```python
from build123d import *

# Parameters (mm, degrees)
F1_DEPTH    = 9.525
F3_DEPTH    = 33.02
F4_T1_DEPTH = 49.53
F6_DEPTH    = 10.16
F7_R        = 3.175
F8_DEPTH    = 25.4
F10_DEPTH   = 25.4


# Not quite as in the source:
# - a fillet or chamfer that OpenCascade refuses, or shapes differently, is made with other operations: its cross-section is extruded or revolved along the edge and cut away or added


with BuildPart() as f1:
    # F0 (on Front) → F1 (new body, symmetric)
    with BuildSketch(Plane.XZ):
        Polygon((-5.715, 0), (0, 0), (0, 1.778), (21.59, 1.778), (21.59, 0), (27.305, 0), (27.305, 4.572), (-5.715, 4.572), align=None)
    extrude(amount=F1_DEPTH, both=True)

    # F2 (on face) → F3 (cut)
    with BuildSketch(Plane.YZ.offset(27.305)):
        Polygon((-2.286, 0), (0, 0), (2.286, 0), (2.286, 1.778), (0, 1.778), (-2.286, 1.778), align=None)
    extrude(amount=-F3_DEPTH, mode=Mode.SUBTRACT)

    # F4: fillet of radius 3.302 on 2 edges, made by hand

    # F4_s2 → F4_t1 (cut)
    with BuildSketch(Plane.YZ.offset(-13.97)):
        with BuildLine():
            ThreePointArc((-6.223, 4.572), (-8.5578665915, 3.6048665915), (-9.525, 1.27))
            Line((-9.525, 1.27), (-9.525, 4.572))
            Line((-9.525, 4.572), (-6.223, 4.572))
        make_face()
        with BuildLine():
            ThreePointArc((9.525, 1.27), (8.5578665915, 3.6048665915), (6.223, 4.572))
            Line((6.223, 4.572), (9.525, 4.572))
            Line((9.525, 4.572), (9.525, 1.27))
        make_face()
    extrude(amount=F4_T1_DEPTH, mode=Mode.SUBTRACT)

    # F5 (on face) → F6 (join)
    with BuildSketch(Plane.XY.offset(4.572)):
        Polygon((-5.715, 3.429), (-5.715, 0), (-5.715, -3.429), (5.969, -3.429), (5.969, 3.429), align=None)
        Polygon((27.305, 0), (27.305, 3.429), (15.621, 3.429), (15.621, -3.429), (27.305, -3.429), align=None)
    extrude(amount=F6_DEPTH)

    # F7 (on face) → F8 (cut)
    with BuildSketch(Plane.XZ.offset(3.429)):
        Polygon((-5.715, 14.732), (-5.715, 8.382), (0.127, 14.732), align=None)
        with Locations((0, 8.382)):
            Circle(F7_R)
    extrude(amount=-F8_DEPTH, mode=Mode.SUBTRACT)

    # F9 (on face) → F10 (cut)
    with BuildSketch(Plane.XZ.offset(3.429)):
        Polygon((27.305, 14.732), (20.955, 14.732), (27.305, 8.382), align=None)
    extrude(amount=-F10_DEPTH, mode=Mode.SUBTRACT)


solid = f1.part
```
Build history of the part. All positions in model axes, mm. A direction names the side the tool comes from. Give positions to 0.01 mm unless a question says otherwise; leave off trailing zeros. Order: outer loops, then holes, each group sorted by start corner. A loop starts at its lowest first (then second) coordinate and runs counter-clockwise, first axis right, second up. Notation, with made-up numbers: M 37,-33 L 77,-33 A26 cw 77,-2 Z; hole C -7.5,8.25 d11. An arc over 180 degrees is marked long. Write item = value, one per line. Start each with the question number.
(1) Probe L1, parallel to X at y = -7.5, z = 1 (3 decimals); L2, parallel to Y at x = 21.5, z = 5; L3, parallel to X at y = 1.5, z = 6.25 (3 decimals). List the from-to ranges inside material, lowest first. Write a range as [from, to].
(2) Slice it at C-C on y = 7.5. Write the cut outline in (x, z) (3 decimals), plus the area to 3 significant figures.
(3) Pin check, flat tips, straight feed: pin 1 Ø1.5 at (x, z) = (7, 4) entering from -Y; pin 2 Ø8 at (x, z) = (22.5, 9.5) entering from -Y; pin 3 Ø3 at (x, z) = (24, 8) entering from +Y. Stop position of each tip, or through.
(4) Slice it at B-B on x = 5. Write the cut outline in (y, z), plus the area to 3 significant figures.
(5) Which spindle directions (+Z, -Z, +X, -X, +Y, -Y) get a long thin tool onto all of the face, cutting with end or side? Do faces 5 (the flat face through (3, 3.429, 11)), 6 (the flat face through (20, -3.429, 10)), 7 (the flat face through (0, 6, 1)), 8 (the flat face through (-3, 2.286, 1)). Say none if no direction does.
(6) Two-plate mould, pull along X, no slides. Class faces 1 (the flat face through (27.305, 0, 3)), 2 (the cylindrical face through (-0.41, -0.05, 11.53)), 3 (the flat face through (24, 9.525, 1)), 4 (the flat face through (21.59, 6, 1)): released by +X, released by -X, zero draft, split by the parting line, or undercut.
(7) Slice it at D-D on x = 22. Write the cut outline in (y, z) (3 decimals), plus the area to 3 significant figures.
(8) Slice it at A-A on z = 13.25. Write the cut outline in (x, y), plus the area to 3 significant figures.
Responses:
q1.L1 = [-5.715, 0], [21.59, 27.305]
q1.L2 = [-3.43, 3.43]
q1.L3 = [-5.715, -2.353], [2.353, 5.969], [15.621, 27.305]
q2.outline = M -5.715,0 L 0,0 L 0,1.778 L 21.59,1.778 L 21.59,0 L 27.305,0 L 27.305,4.315 L -5.715,4.315 Z
q2.area = 104 mm2
q3.pin_1 = -8.87
q3.pin_2 = -3.43
q3.pin_3 = 3.43
q4.outline = M -9.49,1.78 L 9.49,1.78 A3.3 ccw 6.22,4.57 L 3.43,4.57 L 3.43,14.73 L -3.43,14.73 L -3.43,4.57 L -6.22,4.57 A3.3 ccw Z
q4.area = 118 mm2
q5.face_5 = +Z, +X, -X, +Y
q5.face_6 = +Z, +X, -X, -Y
q5.face_7 = -Z, +Y, -Y
q5.face_8 = -Z, +X, -X
q6.face_1 = released by +X
q6.face_2 = undercut
q6.face_3 = zero draft
q6.face_4 = undercut
q7.outline = M -9.525,0 L -2.286,0 L -2.286,1.778 L 2.286,1.778 L 2.286,0 L 9.525,0 L 9.525,1.27 A3.302 ccw 6.223,4.572 L 3.429,4.572 L 3.429,13.687 L -3.429,13.687 L -3.429,4.572 L -6.223,4.572 A3.302 ccw -9.525,1.27 Z
q7.area = 137 mm2
q8.outline = M -1.24,-3.43 L 5.97,-3.43 L 5.97,3.43 L -1.24,3.43 Z; M 15.62,-3.43 L 22.44,-3.43 L 22.44,3.43 L 15.62,3.43 Z
q8.area = 96.2 mm2
